```python
from build123d import *

# Parameters (mm, degrees)
PAD007_DEPTH    = 12
SKETCH017_R     = 1.8
HOLE004_DEPTH   = 15.001
POCKET003_DEPTH = 18.1900462152


with BuildPart() as part:
    # Sketch016 → Pad007 (new body)
    with BuildSketch(Plane.YZ.offset(3)):
        with BuildLine():
            Line((40.1500266983, 43.3493812581), (13.7307513645, 48.919111129))
            ThreePointArc((10.6419298144, 53.6582230111), (11.2048383818, 50.6489511812), (13.7307513645, 48.919111129))
            Line((10.6419298144, 53.6582230111), (11.4670749804, 57.5721897273))
            ThreePointArc((16.2061868626, 60.6610112773), (13.1969150326, 60.0981027099), (11.4670749804, 57.5721897273))
            Line((16.2061868626, 60.6610112773), (42.6254621965, 55.0912814065))
            ThreePointArc((45.7142837465, 50.3521695243), (45.1513751791, 53.3614413543), (42.6254621965, 55.0912814065))
            Line((45.7142837465, 50.3521695243), (44.8891385805, 46.4382028082))
            ThreePointArc((40.1500266983, 43.3493812581), (43.1592985283, 43.9122898256), (44.8891385805, 46.4382028082))
        make_face()
    extrude(amount=PAD007_DEPTH)

    # Sketch017 → Hole004 (cut, through all)
    with BuildSketch(Plane.YZ):
        with Locations((15.9469607926, 54.5837749116)):
            Circle(SKETCH017_R)
        with Locations((40.4092527683, 49.4266176238)):
            Circle(SKETCH017_R)
    extrude(amount=HOLE004_DEPTH, mode=Mode.SUBTRACT)

    # Sketch018 (on ShapeBinder) → Pocket003 (cut, through all)
    with BuildSketch(Plane(origin=(0, 10.4585930571, 49.6089498031), x_dir=(0, 0.978491679, -0.2062862915), z_dir=(0, -0.2062862915, -0.978491679))):
        with BuildLine():
            Line((8.8440839381, 21), (8.8440839381, 11))
            ThreePointArc((8.8440839381, 11), (9.5525813159, 7.7084973779), (11.5525813159, 5))
            Line((11.5525813159, 5), (22.1355865602, 5))
            ThreePointArc((22.1355865602, 5), (24.1355865602, 7.7084973779), (24.8440839381, 11))
            Line((24.8440839381, 11), (24.8440839381, 21))
            Line((24.8440839381, 21), (8.8440839381, 21))
        make_face()
    extrude(amount=-POCKET003_DEPTH, mode=Mode.SUBTRACT)


solid = part.part
```
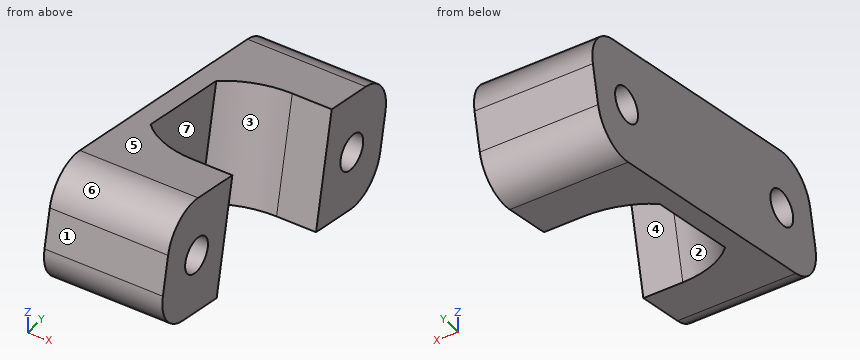
Design review of the part built by this model. Coordinates are the model's own, in mm. Face numbers are marked on the shaded views. A direction names the side the tool comes from. Round coordinates to 2 decimals unless told otherwise and drop trailing zeros. Write each loop counter-clockwise with the first axis right and the second up, starting at its lowest first coordinate (ties: lowest second). Pieces come first, ordered by that corner, then holes.
Item 1: The part is to be moulded in two halves that separate along Y. For the marked faces 4, 5, 6 and 7, say which applies: +Y half, -Y half, draft (parallel to the pull), parting line (faces both ways), or undercut.
Item 2: We need section C-C on x = 4.25. Write out the cut boundary in (y, z), and give its area (3 significant figures).
Item 3: We need section A-A on x = 13.75. Write out the cut boundary in (y, z), and give its area (3 significant figures).
Item 4: For the marked faces 1, 2 and 3, list the 3-axis set-ups (+Z, -Z, +X, -X, +Y, -Y) from which the entire face can be reached by the end or side of a thin tool; tool diameter is ignored.
Item 5: We need section B-B on x = 10. Write out the cut boundary in (y, z), and give its area (3 significant figures).
Item 6: Clearance check with flat-ended pins moving along their axes: pin 1 Ø6 at (x, y) = (11, 24.5) entering from +Z; pin 2 Ø1 at (x, z) = (6, 50) entering from -Y; pin 3 Ø4 at (x, z) = (4.5, 58) entering from -Y. State where each tip first meets the part, or that it passes through.
Item 7: We need section D-D on y = 27. Write out the cut boundary in (x, z), and give its area (3 significant figures).
Item 8: For probe 1 along Y at (x, z) = (5.5, 49.25); probe 2 along Y at (x, z) = (8, 50); probe 3 along X at (y, z) = (22.5, 49.5), list the stretches that pass through material, from the lowest coordinate up.
Returned:
1. face 4: undercut
1. face 5: +Y half
1. face 6: parting line
1. face 7: undercut
2. outline: (10.64, 53.66) arc R4 ccw to (13.73, 48.92) - (40.15, 43.35) arc R4 ccw to (44.89, 46.44) - (45.71, 50.35) arc R4 ccw to (42.63, 55.09) - (16.21, 60.66) arc R4 ccw to (11.47, 57.57) - close; hole circle Ø3.6 at (15.95, 54.58); hole circle Ø3.6 at (40.41, 49.43)
2. area: 386 mm2
3. outline: (10.64, 53.66) arc R4 ccw to (13.73, 48.92) - (19.11, 47.78) - (21.59, 59.53) - (16.21, 60.66) arc R4 ccw to (11.47, 57.57) - close; (34.77, 44.48) - (40.15, 43.35) arc R4 ccw to (44.89, 46.44) - (45.71, 50.35) arc R4 ccw to (42.63, 55.09) - (37.24, 56.23) - close; hole circle Ø3.6 at (15.95, 54.58); hole circle Ø3.6 at (40.41, 49.43)
3. area: 194 mm2
4. face 1: +Z, +X, -X, -Y
4. face 2: -Z, +X
4. face 3: +Z, +X
5. outline: (10.64, 53.66) arc R4 ccw to (13.73, 48.92) - (19.17, 47.77) - (21.65, 59.51) - (16.21, 60.66) arc R4 ccw to (11.47, 57.57) - close; (34.71, 44.5) - (40.15, 43.35) arc R4 ccw to (44.89, 46.44) - (45.71, 50.35) arc R4 ccw to (42.63, 55.09) - (37.18, 56.24) - close; hole circle Ø3.6 at (15.95, 54.58); hole circle Ø3.6 at (40.41, 49.43)
5. area: 195 mm2
6. pin 1: stops at z = 59.54
6. pin 2: stops at y = 11.31
6. pin 3: stops at y = 11.14
7. outline: (3, 46.12) - (5, 46.12) - (5, 58.39) - (3, 58.39) - close
7. area: 24.5 mm2
8. probe 1: y = 12.78 to 21.66, 33.53 to 38.62, 42.2 to 45.48
8. probe 2: y = 11.73 to 20.18, 35.33 to 38.7, 42.12 to 45.64
8. probe 3: x = 3 to 5
